Geometry: see drawing. Coordinates: mm, zero at the bounding-box minimum. A direction names the side the tool comes from. Coordinates: 2 decimals unless noted, no trailing zeros. Loops run counter-clockwise (first coordinate to the right, second up) from the corner with the lowest first, then second, coordinate; pieces in that order, holes last. Notation, with made-up numbers: (19, -17.75) - (56, -17.75) arc R18 cw to (56, 9.25) - close; hole circle Ø1 at (-13, 76). An arc over 180 degrees is marked (long way). Use one line per item in the form item = value.
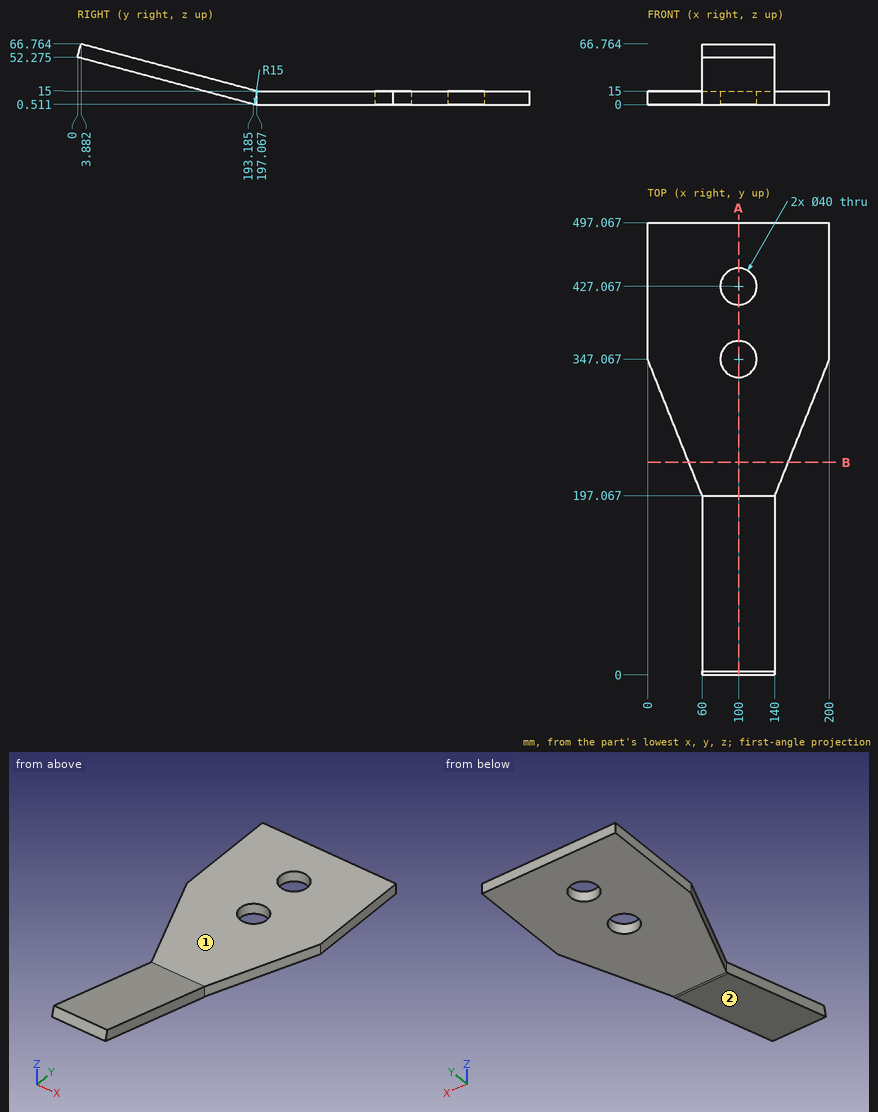
Q1. Set-up query: the marked faces 1 and 2. Return all of +Z, -Z, +X, -X, +Y, -Y with unobstructed straight access to the full face (end or side cutting, diameter ignored); none if empty.
Check values:
face_1 = +Z, +X, -X, +Y
face_2 = -Z, +X, -X, -Y
Q2. First-contact query: P1, Ø4, axis at x = 57.5, z = 10, coming from the -Y side (1 decimal); P2, Ø1, axis at x = 101.5, y = 232, coming from the +Z side. Flat tips, straight axial feed; report the tip coordinate or a pass-through.
Check values:
P1 = 198.3
P2 = 15
Q3. Ray query, line 1 along Z through (x, y) = (171.5, 349); line 2 along X through (y, z) = (134, 29.5); line 3 along Z through (x, y) = (116, 134.5) (1 decimal). Return the intervals inside material, ascending. Write a range as [from, to].
Check values:
line_1 = [0, 15]
line_2 = [60, 140]
line_3 = [16.2, 31.8]
Q4. Cut plane B-B, the plane y = 233.5. Return loops of the section in (x, z), then the cut area to 3 significant figures.
Check values:
outline = (45.43, 0) - (154.57, 0) - (154.57, 15) - (45.43, 15) - close
area = 1,640 mm²
Q5. Cut plane A-A, the plane x = 100. Return loops of the section in (y, z) (1 decimal), then the cut area to 3 significant figures.
Check values:
outline = (0, 52.3) - (193.2, 0.5) arc R15 ccw to (197.1, 0) - (327.1, 0) - (327.1, 15) - (197.1, 15) - (3.9, 66.8) - close; (367.1, 0) - (407.1, 0) - (407.1, 15) - (367.1, 15) - close; (447.1, 0) - (497.1, 0) - (497.1, 15) - (447.1, 15) - close
area = 6,330 mm²
